Could you check a few things on this model? Use its own coordinates, in mm. Face numbers are marked on the shaded views. A direction names the side the tool comes from. Round coordinates to 2 decimals unless told otherwise and drop trailing zeros. Write each loop counter-clockwise with the first axis right and the second up, starting at its lowest first coordinate (ties: lowest second). Pieces come first, ordered by that corner, then holes. Notation, with made-up numbers: (44, 55) -> (67, 55) arc R15 cw to (67, 63) -> close; hole circle Ø7 at (23, -3). An arc over 180 degrees is marked (long way). Answer in a Markdown table with one row per item. Add a question column.
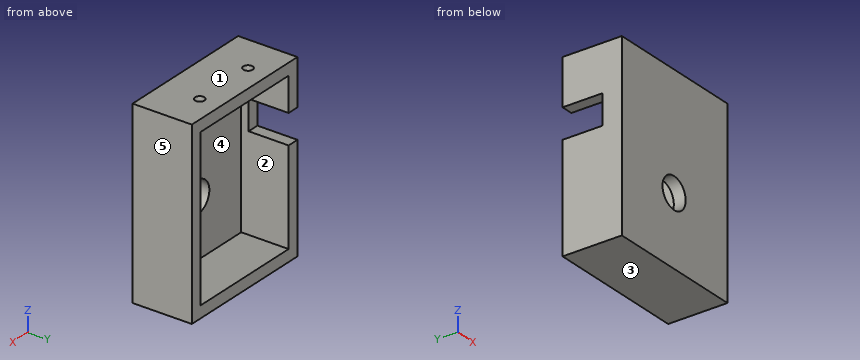
Autodesk Inventor part; units mm, degrees
ref_plane "YZ Plane" through (0, 0, 0) normal (1, 0, 0) x (0, 1, 0)
ref_plane "XZ Plane" through (0, 0, 0) normal (0, 1, 0) x (-1, 0, 0)
ref_plane "XY Plane" through (0, 0, 0) normal (0, 0, 1) x (1, 0, 0)
sketch "Sketch1" plane through (0, 0, 0) normal (0, 1, 0) x (-1, 0, 0)
  line L0 (0, 0) -> (-50.673, 0)
  line L1 (-50.673, 0) -> (-50.673, -67.818)
  line L2 (-50.673, -67.818) -> (0, -67.818)
  line L3 (0, -67.818) -> (0, 0)
  line L4 (5.08, -72.898) -> (-55.753, -72.898)
  line L5 (-55.753, -72.898) -> (-55.753, 5.08)
  line L6 (-55.753, 5.08) -> (5.08, 5.08)
  line L7 (5.08, 5.08) -> (5.08, -72.898)
  circle A0 centre (-25.019, -43.2562) radius 6.6675
  circle A1 centre (34.7838, -26.9997) radius 2.286
  dimension "d0" = 50.673
  dimension "d1" = 67.818
  dimension "d2" = 5.08
  dimension "d11" = 13.335
  dimension "d14" = 4.572
extrude "Extrusion1" add sketch "Sketch1" along normal blind 20.32 and the other way blind 5.08 contours L4 L5 L6 L7
extrude "Extrusion2" add sketch "Sketch1" against normal blind 5.08 contours L3 L2 L1 L0 | A0
extrude "Extrusion3" cut sketch "Sketch1" against normal blind 127 contours A0
sketch "Sketch2" plane through (-5.08, -5.08, 5.08) normal (-1, 0, 0) x (0, 0, 1)
  line L0 (0, 25.4) -> (-19.685, 25.4)
  line L1 (-77.978, 25.4) -> (0, 25.4)
  line L2 (-19.685, 25.4) -> (-19.685, 8.255)
  line L3 (-5.08, 5.08) -> (-72.898, 5.08)
  line L4 (-19.685, 8.255) -> (-32.385, 8.255)
  line L5 (-32.385, 8.255) -> (-32.385, 25.4)
  line L6 (-19.685, 25.4) -> (-32.385, 25.4)
  dimension "d15" = 19.685
  dimension "d16" = 17.145
  dimension "d17" = 12.7
extrude "Extrusion4" cut sketch "Sketch2" against normal blind 25.4
sketch "Sketch5" plane through (-5.08, 20.32, 5.08) normal (0, 0, 1) x (1, 0, 0)
  line L0 (16.51, 0) -> (16.51, -8.89)
  line L1 (0, 0) -> (0, -25.4)
  line L2 (60.833, 0) -> (44.323, 0)
  line L3 (0, 0) -> (60.833, 0)
  line L4 (44.323, 0) -> (44.323, -8.89)
  circle A0 centre (44.323, -8.89) radius 2.032
  circle A1 centre (16.51, -8.89) radius 2.032
  point P0 (5.08, -20.32)
  point P1 (16.51, -0.0329)
  dimension "d21" = 8.89
  dimension "d22" = 16.51
  dimension "d23" = 16.51
  dimension "d24" = 8.89
  dimension "d25" = 4.064
  dimension "d26" = 4.064
extrude "Extrusion5" cut sketch "Sketch5" against normal blind 25.4
properties part number "BH_Engineering Club Autonomous Car_Encoder Holder"
(1) Suppose I cut it at D-D, the plane z = -25.5. Please give me the cut outline in (x, y) (3 decimals).
(2) On a 3-axis mill with a long thin cutter (end or side, diameter ignored), from which of +Z, -Z, +X, -X, +Y, -Y can I reach the whole of each face in a straight line? I mean the marked faces 1 and 2. Say none if no direction works.
(3) Suppose I cut it at A-A, the plane x = 11.43. Please give me the cut outline in (y, z), then the cut area to 3 significant figures.
(4) I need wall thicknesses on L1, parallel to X at y = 11.43, z = 1.4 (3 decimals); L2, parallel to Z at x = 12, y = 0.25; L3, parallel to Z at x = -0.5, y = 5 (3 decimals). Which ranges of each line are inside material? Lowest first, please.
(5) Suppose I cut it at B-B, the plane y = 11.43. Please give me the cut outline in (x, z) (3 decimals).
(6) If we mould it in two halves opening along X, with no side actions, what happens to the marked faces 3, 4 and 5? For each: pulls with the +X half, pulls with the -X half, needs draft (parallel to the pull), parting line crosses it, or undercut.
(7) Suppose I cut it at C-C, the plane y = 1. Please give me the cut outline in (x, z).
(8) For P1, Ø2, axis at x = 5.5, z = -23.5, coming from the +Y side; P2, Ø8, axis at x = 25.02, z = -43.26, coming from the +Y side; P3, Ø5.5, axis at x = -3, z = -19.5, coming from the +Y side (3 decimals); P4, Ø3.5, axis at x = 39.243, y = 11.43, coming from the +Z side, each with a flat end and sliding along its axis, tell me the tip position at first contact or that it passes through.
Response:
| question | item | result |
|---|---|---|
| 1 | outline | (-5.08, -5.08) -> (55.753, -5.08) -> (55.753, 20.32) -> (50.673, 20.32) -> (50.673, 0) -> (0, 0) -> (0, 3.175) -> (-5.08, 3.175) -> close |
| 2 | face 1 | +Z, +X, -X, +Y, -Y |
| 2 | face 2 | +Y |
| 3 | outline | (-5.08, -72.9) -> (20.32, -72.9) -> (20.32, -67.82) -> (0, -67.82) -> (0, 0) -> (9.4, 0) -> (9.4, 5.08) -> (-5.08, 5.08) -> close; (13.46, 0) -> (20.32, 0) -> (20.32, 5.08) -> (13.46, 5.08) -> close |
| 3 | area | 582 mm² |
| 4 | L1 | -5.08 to 9.398, 13.462 to 37.211, 41.275 to 55.753 |
| 4 | L2 | -72.9 to -67.82, 0 to 5.08 |
| 4 | L3 | -72.898 to -27.305, -14.605 to 5.08 |
| 5 | outline | (-5.08, -72.898) -> (55.753, -72.898) -> (55.753, 5.08) -> (41.275, 5.08) -> (41.275, 0) -> (50.673, 0) -> (50.673, -67.818) -> (0, -67.818) -> (0, -27.305) -> (-5.08, -27.305) -> close; (-5.08, -14.605) -> (0, -14.605) -> (0, 0) -> (9.398, 0) -> (9.398, 5.08) -> (-5.08, 5.08) -> close; (13.462, 0) -> (37.211, 0) -> (37.211, 5.08) -> (13.462, 5.08) -> close |
| 6 | face 3 | needs draft |
| 6 | face 4 | undercut |
| 6 | face 5 | pulls with the +X half |
| 7 | outline | (-5.08, -72.9) -> (55.75, -72.9) -> (55.75, 5.08) -> (-5.08, 5.08) -> close; hole (0, -67.82) -> (50.67, -67.82) -> (50.67, 0) -> (0, 0) -> close |
| 8 | P1 | y = 0 |
| 8 | P2 | through |
| 8 | P3 | y = 3.175 |
| 8 | P4 | z = -67.82 |
